Geometry: see drawing. Coordinates: mm, zero at the bounding-box minimum. Give positions to 0.01 mm unless a question says otherwise; leave off trailing zeros. Order: outer loops, then holes, each group sorted by start corner. A loop starts at its lowest first (then second) coordinate and runs counter-clockwise, first axis right, second up. Notation, with made-up numbers: M -38.5,0 L -26.5,0 A31 ccw -26.5,27 Z; hole C 33,77.5 d7. An arc over 180 degrees is marked long. Answer as a JSON object with one key per item and string values. Group by question number.
1. Material intervals for L1, parallel to X at y = 1.5, z = 68.5; L2, parallel to X at y = 0.5, z = 32.5; L3, parallel to Z at x = 268.5, y = 3, sorted ascending. Write a range as [from, to].
2. Pin query (flat end, axial travel): P1, Ø1.9, axis at y = 4.5, z = 4.5, coming from the +X side. Return the tip coordinate at first contact, or that it passes through.
3. Section query B-B (x = 174.5). Output: boundary loops of the cut face in (y, z), plus the area to 3 significant figures.
4. Section query D-D (z = 215). Output: boundary loops of the cut face in (x, y), plus the area to 3 significant figures.
5. Section query A-A (z = 87.63). Output: boundary loops of the cut face in (x, y), plus the area to 3 significant figures.
6. Section query C-C (y = 3.25). Count the separate pieces of the cut face and the enclosed holes in it, plus the area to 3 significant figures.
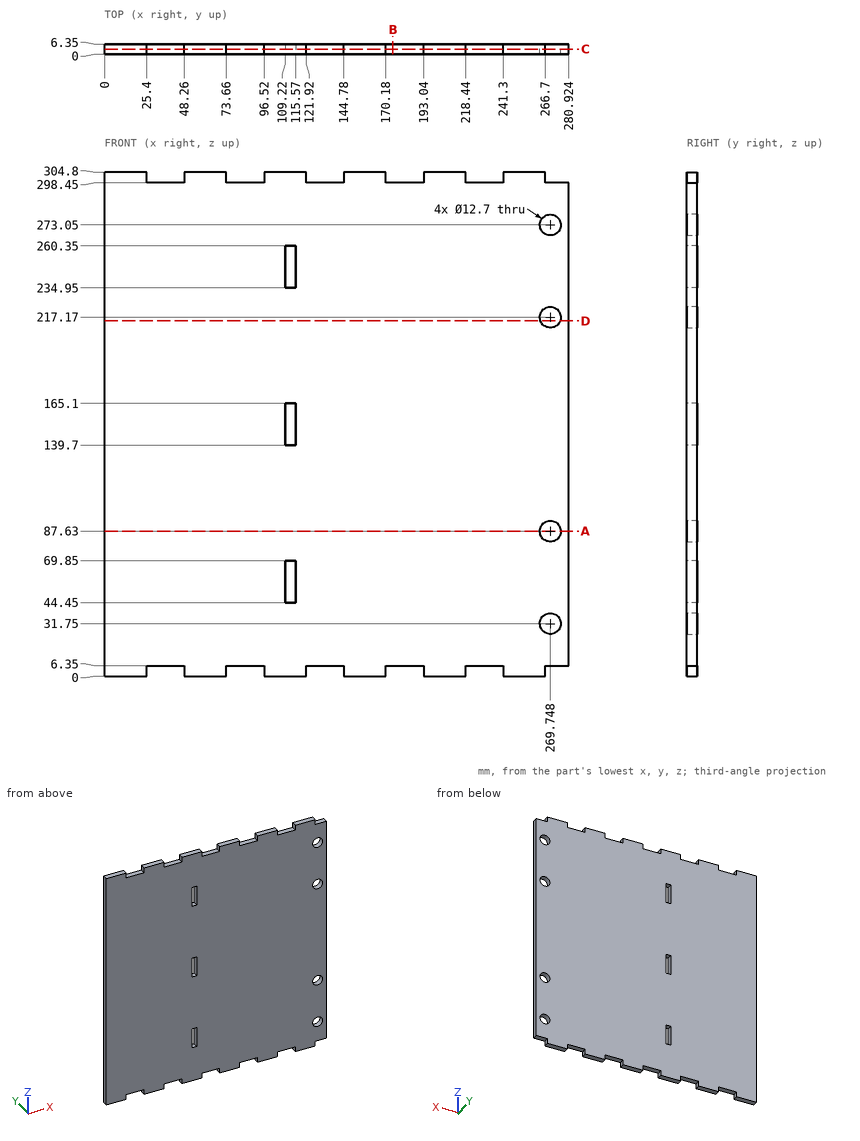
Answer sheet:
{
 "1": {"L1": "[0, 109.22], [115.57, 280.92]", "L2": "[0, 263.44], [276.05, 280.92]", "L3": "[6.35, 25.52], [37.98, 81.4], [93.86, 210.94], [223.4, 266.82], [279.28, 298.45]"},
 "2": {"P1": "x = 266.7"},
 "3": {"outline": "M 0,6.35 L 6.35,6.35 L 6.35,298.45 L 0,298.45 Z", "area": "1,850 mm^2"},
 "4": {"outline": "M 0,0 L 263.78,0 L 263.78,6.35 L 0,6.35 Z; M 275.72,0 L 280.92,0 L 280.92,6.35 L 275.72,6.35 Z", "area": "1,710 mm^2"},
 "5": {"outline": "M 0,0 L 263.4,0 L 263.4,6.35 L 0,6.35 Z; M 276.1,0 L 280.92,0 L 280.92,6.35 L 276.1,6.35 Z", "area": "1,700 mm^2"},
 "6": {"separate pieces": "1", "enclosed holes": "7", "area": "83,000 mm^2"}
}
